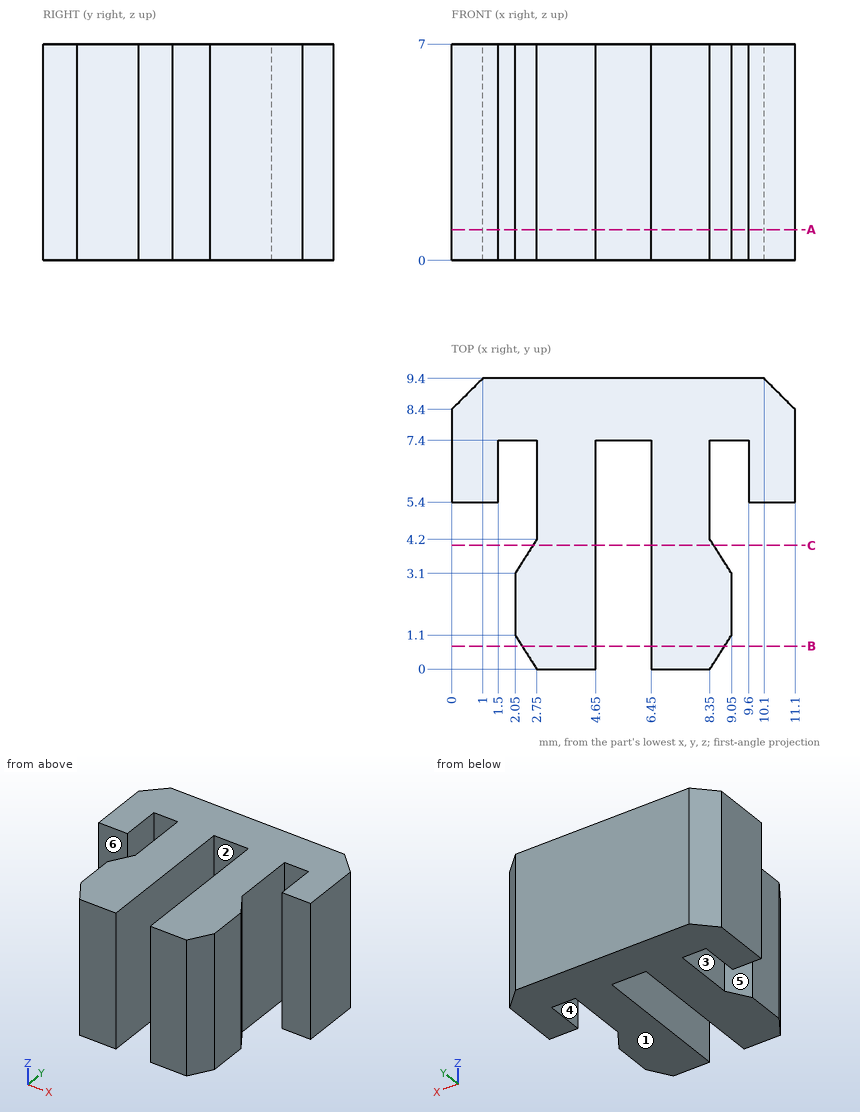
The drawing under review shows one solid part. Ordinate dimensions are in mm from its lowest x, y, z. A direction names the side the tool comes from. Give positions to 0.01 mm unless a question says otherwise; leave off trailing zeros. Write each loop counter-clockwise with the first axis right and the second up, starting at its lowest first coordinate (ties: lowest second). Pieces come first, ordered by that corner, then holes. Notation, with made-up numbers: (-1, 50) -> (48, 50) arc R11 ccw to (48, 69) -> close; hole circle Ø2 at (81, -12). An arc over 180 degrees is marked (long way). Answer in a Markdown table with one row per item.
(1) Consider section A-A (z = 1). State the section outline as (x, y) points.
Results:
| item | result |
|---|---|
| outline | (0, 5.4) -> (1.5, 5.4) -> (1.5, 7.4) -> (2.75, 7.4) -> (2.75, 4.2) -> (2.05, 3.1) -> (2.05, 1.1) -> (2.75, 0) -> (4.65, 0) -> (4.65, 7.4) -> (6.45, 7.4) -> (6.45, 0) -> (8.35, 0) -> (9.05, 1.1) -> (9.05, 3.1) -> (8.35, 4.2) -> (8.35, 7.4) -> (9.6, 7.4) -> (9.6, 5.4) -> (11.1, 5.4) -> (11.1, 8.4) -> (10.1, 9.4) -> (1, 9.4) -> (0, 8.4) -> close |
(2) To check wall thickness, follow probe 1 along X at (y, z) = (7.25, 5); probe 2 along X at (y, z) = (5, 1.5); probe 3 along X at (y, z) = (2, 2.5). State the ranges of each line that lie inside material, in increasing order.
Results:
| item | result |
|---|---|
| probe 1 | 0 to 1.5, 2.75 to 4.65, 6.45 to 8.35, 9.6 to 11.1 |
| probe 2 | 2.75 to 4.65, 6.45 to 8.35 |
| probe 3 | 2.05 to 4.65, 6.45 to 9.05 |
(3) Consider section C-C (y = 4). State the section outline as (x, z) points, then the cut area to 3 significant figures.
Results:
| item | result |
|---|---|
| outline | (2.62, 0) -> (4.65, 0) -> (4.65, 7) -> (2.62, 7) -> close; (6.45, 0) -> (8.48, 0) -> (8.48, 7) -> (6.45, 7) -> close |
| area | 28.4 mm2 |
(4) Mouldability with a two-part tool opening along Y and no side actions: class the marked faces 1, 2 and 3 as +Y half, -Y half, draft (parallel to the pull), parting line (faces both ways), or undercut.
Results:
| item | result |
|---|---|
| face 1 | draft |
| face 2 | -Y half |
| face 3 | undercut |
(5) Clearance check with flat-ended pins moving along their axes: pin 1 (2 mm diameter, centred on y = 2, z = 3, fed in from +X); pin 2 (1.5 mm diameter, centred on x = 1.5, z = 5, fed in from -Y); pin 3 (1.6 mm diameter, centred on x = 1, z = 4, fed in from -Y). State where each tip first meets the part, or that it passes through.
Results:
| item | result |
|---|---|
| pin 1 | x = 9.05 |
| pin 2 | y = 0.79 |
| pin 3 | y = 5.4 |
(6) For the marked faces 4, 5 and 6, list the 3-axis set-ups (+Z, -Z, +X, -X, +Y, -Y) from which the entire face can be reached by the end or side of a thin tool; tool diameter is ignored.
Results:
| item | result |
|---|---|
| face 4 | +Z, -Z, -Y |
| face 5 | +Z, -Z, -X |
| face 6 | +Z, -Z, -X, -Y |
(7) Consider section B-B (y = 0.75). State the section outline as (x, z) points, then the cut area to 3 significant figures.
Results:
| item | result |
|---|---|
| outline | (2.27, 0) -> (4.65, 0) -> (4.65, 7) -> (2.27, 7) -> close; (6.45, 0) -> (8.83, 0) -> (8.83, 7) -> (6.45, 7) -> close |
| area | 33.3 mm2 |
